from build123d import *

# Parameters (mm, degrees)
BOSS_EXTRU_1_START = -10
BOSS_EXTRU_1_DEPTH = 2
BOSS_EXTRU_2_START = -12
BOSS_EXTRU_2_DEPTH = 20
BOSS_EXTRU_3_START = -32
ESQUISSE3_4_W      = 45
ESQUISSE3_4_H      = 57
BOSS_EXTRU_3_DEPTH = 2
BOSS_EXTRU_4_DEPTH = 2
BOSS_EXTRU_5_DEPTH = 94


with BuildPart() as part:
    # Esquisse3 → Boss.-Extru.1 (new body)
    with BuildSketch(Plane(origin=(0, 0, 66.961524227), x_dir=(-1, 0, 0), z_dir=(0, 0, -1)).offset(BOSS_EXTRU_1_START)):
        Polygon((47, -2), (47, 92), (-47, 92), (-47, -2), (-24.5, -2), (-24.5, 57), (24.5, 57), (24.5, -2), align=None)
        Polygon((22.5, -2), (24.5, -2), (24.5, 57), (-24.5, 57), (-24.5, -2), (-22.5, -2), (-22.5, 55), (22.5, 55), align=None)
    extrude(amount=-BOSS_EXTRU_1_DEPTH)

    # Esquisse3<3> → Boss.-Extru.2 (add)
    with BuildSketch(Plane(origin=(0, 0, 66.961524227), x_dir=(-1, 0, 0), z_dir=(0, 0, -1)).offset(BOSS_EXTRU_2_START)):
        Polygon((22.5, -2), (24.5, -2), (24.5, 57), (-24.5, 57), (-24.5, -2), (-22.5, -2), (-22.5, 55), (22.5, 55), align=None)
    extrude(amount=-BOSS_EXTRU_2_DEPTH)

    # Esquisse3<4> → Boss.-Extru.3 (add)
    with BuildSketch(Plane(origin=(0, 0, 66.961524227), x_dir=(-1, 0, 0), z_dir=(0, 0, -1)).offset(BOSS_EXTRU_3_START)):
        with Locations((0, 26.5)):
            Rectangle(ESQUISSE3_4_W, ESQUISSE3_4_H)
    extrude(amount=BOSS_EXTRU_3_DEPTH)

    # Esquisse4 → Boss.-Extru.4 (add)
    with BuildSketch(Plane(origin=(0, 92, 0), x_dir=(1, 0, 0), z_dir=(0, 1, 0))):
        with BuildLine():
            Line((-45, -27.041634566), (-45, -76.961524227))
            Line((-45, -76.961524227), (45, -76.961524227))
            Line((45, -76.961524227), (45, -27.041634566))
            ThreePointArc((45, -27.041634566), (33.944628417, -40.050121119), (19.3, -48.823764705))
            Line((19.3, -48.823764705), (19.3, -61.001524227))
            Line((19.3, -61.001524227), (-19.3, -61.001524227))
            Line((-19.3, -61.001524227), (-19.3, -48.823764705))
            ThreePointArc((-19.3, -48.823764705), (-33.944628417, -40.050121119), (-45, -27.041634566))
        make_face()
    extrude(amount=-BOSS_EXTRU_4_DEPTH)

    # Esquisse4<3> → Boss.-Extru.5 (add)
    with BuildSketch(Plane(origin=(0, 92, 0), x_dir=(1, 0, 0), z_dir=(0, 1, 0))):
        with BuildLine():
            Line((45, -27.041634566), (45, -76.961524227))
            Line((45, -76.961524227), (47, -76.961524227))
            Line((47, -76.961524227), (47, -23.393375131))
            ThreePointArc((47, -23.393375131), (46.036153719, -25.237324557), (45, -27.041634566))
        make_face()
        with BuildLine():
            ThreePointArc((-47, -23.393375131), (-46.036153719, -25.237324557), (-45, -27.041634566))
            Line((-45, -27.041634566), (-45, -76.961524227))
            Line((-45, -76.961524227), (-47, -76.961524227))
            Line((-47, -76.961524227), (-47, -23.393375131))
        make_face()
    extrude(amount=-BOSS_EXTRU_5_DEPTH)


solid = part.part
The model under review builds one solid part; all positions refer to its coordinate system, in mm. A direction names the side the tool comes from. Round coordinates to 2 decimals unless told otherwise and drop trailing zeros. Order: outer loops, then holes, each group sorted by start corner. A loop starts at its lowest first (then second) coordinate and runs counter-clockwise, first axis right, second up. Notation, with made-up numbers: (42, 78.25) -> (46, 78.25) arc R18 ccw to (46, 94.25) -> close; hole circle Ø7 at (61, 15). An arc over 180 degrees is marked (long way). Use CSV: the item, a comma, the result in double quotes. Start each with the question number.
(1) Insertion check: pin 1 (10 mm diameter, centred on y = 19.5, z = 92.5, fed in from -X); pin 2 (12 mm diameter, centred on x = -16.5, y = 81, fed in from +Z); pin 3 (25 mm diameter, centred on x = -15.5, z = 54, fed in from -Y); pin 4 (8 mm diameter, centred on x = 28, z = 39.5, fed in from -Y). Each pin has a flat end and moves straight along its axis. Give the tip position at first contact, or say it passes through.
(2) Consider section C-C on x = -6. Write out the cut boundary in (y, z), and give its area (3 significant figures).
(3) Wall thickness on probe 1 along X at (y, z) = (50, 68); probe 2 along X at (y, z) = (11.5, 88.5); probe 3 along Z at (x, y) = (30.5, 58.5): over which ranges is each line inside the solid? List them lowest first. Write a range as from..to.
(4) Consider section B-B on y = 73.5. Write out the cut boundary in (x, z), and give its area (3 significant figures).
(5) Consider section D-D on z = 91. Write out the cut boundary in (x, y).
(6) Consider section A-A on z = 51.5. Write out the cut boundary in (x, y), and give its area (3 significant figures).
(7) Tool access review of faces 4 (the face through (47, 46, 52)), 5 (the face through (24.5, 28, 89)), 6 (the face through (0, 57, 89)), 7 (the face through (-24.5, 27, 89)), 8 (the face through (1, 65, 76.962)): name each direction out of +Z, -Z, +X, -X, +Y, -Y from which nothing blocks a thin tool from reaching the whole face with its end or side.
(8) Mouldability with a two-part tool opening along X and no side actions: class faces 1 (the face through (-22.5, 27, 87)), 2 (the face through (-1, 92, 63)), 3 (the face through (-47, 44, 51)) as pulls with the +X half, pulls with the -X half, needs draft (parallel to the pull), parting line crosses it, or undercut.
Responses:
1,pin 1,"x = -24.5"
1,pin 2,"z = 78.96"
1,pin 3,"y = 90"
1,pin 4,"through"
2,outline,"(-2, 96.96) -> (55, 96.96) -> (55, 76.96) -> (90, 76.96) -> (90, 61) -> (92, 61) -> (92, 78.96) -> (57, 78.96) -> (57, 98.96) -> (-2, 98.96) -> close"
2,area,"260 mm²"
3,probe 1,"-47..-45, 45..47"
3,probe 2,"-24.5..-22.5, 22.5..24.5"
3,probe 3,"76.96..78.96"
4,outline,"(-47, 23.39) arc R52.5 cw to (-45, 27.04) -> (-45, 76.96) -> (45, 76.96) -> (45, 27.04) arc R52.5 cw to (47, 23.39) -> (47, 78.96) -> (-47, 78.96) -> close"
4,area,"395 mm²"
5,outline,"(-24.5, -2) -> (-22.5, -2) -> (-22.5, 55) -> (22.5, 55) -> (22.5, -2) -> (24.5, -2) -> (24.5, 57) -> (-24.5, 57) -> close"
6,outline,"(-47, -2) -> (-45, -2) -> (-45, 90) -> (-19.3, 90) -> (-19.3, 92) -> (-47, 92) -> close; (19.3, 90) -> (45, 90) -> (45, -2) -> (47, -2) -> (47, 92) -> (19.3, 92) -> close"
6,area,"479 mm²"
7,face 4,"+Z, -Z, +X, +Y, -Y"
7,face 5,"+Z, +X, +Y, -Y"
7,face 6,"+Z, +X, -X, +Y"
7,face 7,"+Z, -X, +Y, -Y"
7,face 8,"-Z, -Y"
8,face 1,"undercut"
8,face 2,"needs draft"
8,face 3,"pulls with the -X half"
